CAD build for the part. Positions are in the model's coordinates, mm. A direction names the side the tool comes from. Give positions to 0.01 mm unless a question says otherwise; leave off trailing zeros. Order: outer loops, then holes, each group sorted by start corner. A loop starts at its lowest first (then second) coordinate and runs counter-clockwise, first axis right, second up. Notation, with made-up numbers: M 80,80.5 L 133,80.5 A33 ccw 133,118.5 Z; hole C 31.5,50 d3. An arc over 180 degrees is marked long. Put each result on its own line as item: value. Start each with the question number.
1) Cut at B-B (y = -32). Write the cut outline in (x, z).
2) Cut at C-C (x = 6). Write the cut outline in (y, z), and give its area (3 significant figures).
3) Drill centre lines: line 1 (Y direction, x = 0, z = 1.6); line 2 (Y direction, x = 0, z = 6.45); line 3 (Y direction, x = -38.9, z = 3.6). Where is each one in solid material? Low to high. Write a range as [from, to].
4) Two-plate mould, pull along Z, no slides. Class faces 1 (the face through (-19.43, 0.22, 11.4)), 2 (the face through (-20.6, 0.32, 8.57)), 3 (the face through (0, -34, 2)): released by +Z, released by -Z, zero draft, split by the parting line, or undercut.
5) Cut at A-A (x = 38.9). Write the cut outline in (y, z), and give its area (3 significant figures).
6) Pin check, flat tips, straight feed: pin 1 (1.5 mm diameter, centred on y = -9.5, z = 20, fed in from +X); pin 2 (7.5 mm diameter, centred on x = -1.5, y = 0, fed in from -Z); pin 3 (10.5 mm diameter, centred on x = 0, y = -32, fed in from +Z); pin 4 (9 mm diameter, centred on x = 0.5, y = -30.5, fed in from +Z). Stop position of each tip, or through.
7) Tool access for faces 4 (the face through (0, 25, 15)), 5 (the face through (-10, 0, 22)), 6 (the face through (-1.708, -3.015, 2.465)): list every direction of +Z, -Z, +X, -X, +Y, -Y with a clear straight run to the whole face (end or side of a thin tool).
8) Cut at D-D (x = -24). Write the cut outline in (y, z), and give its area (3 significant figures).
```python
from build123d import *

# Parameters (mm, degrees)
SKETCH1_W           = 93.8
SKETCH1_H           = 80
BOSS_EXTRUDE1_DEPTH = 8
SKETCH2_W           = 40
SKETCH2_H           = 50
BOSS_EXTRUDE2_DEPTH = 15
SKETCH4_R           = 2
CUT_EXTRUDE2_DEPTH  = 66.792172787
CUT_EXTRUDE3_DEPTH  = 5
SKETCH7_R           = 2
CUT_EXTRUDE4_DEPTH  = 20
SKETCH8_R           = 4
CUT_EXTRUDE5_DEPTH  = 3
CUT_EXTRUDE6_DEPTH  = 82.268751682
SKETCH10_W          = 3
SKETCH10_H          = 50
CUT_EXTRUDE7_DEPTH  = 2
FILLET2_R           = 2


with BuildPart() as part:
    # Sketch1 → Boss-Extrude1 (new body)
    with BuildSketch(Plane.XY):
        Rectangle(SKETCH1_W, SKETCH1_H)
    extrude(amount=BOSS_EXTRUDE1_DEPTH)

    # Sketch2 → Boss-Extrude2 (add)
    with BuildSketch(Plane.XY.offset(8)):
        Rectangle(SKETCH2_W, SKETCH2_H)
    extrude(amount=BOSS_EXTRUDE2_DEPTH)

    # Sketch4 → Cut-Extrude2 (cut, through all)
    with BuildSketch(Plane(origin=(0, 0, 0), x_dir=(-1, 0, 0), z_dir=(0, 0, -1))):
        with Locations((0, -32)):
            Circle(SKETCH4_R)
        with Locations((0, 32)):
            Circle(SKETCH4_R)
        with Locations((38.9, 0)):
            Circle(SKETCH4_R)
        with Locations((-38.9, 0)):
            Circle(SKETCH4_R)
    extrude(amount=-CUT_EXTRUDE2_DEPTH, mode=Mode.SUBTRACT)

    # Sketch5 → Cut-Extrude3 (cut)
    with BuildSketch(Plane(origin=(0, 0, 0), x_dir=(-1, 0, 0), z_dir=(0, 0, -1))):
        Polygon((0, 4.001037365), (-3.465, 2.000518683), (-3.465, -2.000518683), (0, -4.001037365), (3.465, -2.000518683), (3.465, 2.000518683), align=None)
    extrude(amount=-CUT_EXTRUDE3_DEPTH, mode=Mode.SUBTRACT)

    # Sketch7 → Cut-Extrude4 (cut)
    with BuildSketch(Plane(origin=(0, 0, 5), x_dir=(-1, 0, 0), z_dir=(0, 0, -1))):
        Circle(SKETCH7_R)
    extrude(amount=-CUT_EXTRUDE4_DEPTH, mode=Mode.SUBTRACT)

    # Sketch8 → Cut-Extrude5 (cut)
    with BuildSketch(Plane.XY.offset(8)):
        with Locations((0, 32)):
            Circle(SKETCH8_R)
        with Locations((38.9, 0)):
            Circle(SKETCH8_R)
        with Locations((0, -32)):
            Circle(SKETCH8_R)
        with Locations((-38.9, 0)):
            Circle(SKETCH8_R)
    extrude(amount=-CUT_EXTRUDE5_DEPTH, mode=Mode.SUBTRACT)

    # Sketch9 → Cut-Extrude6 (cut, through all)
    with BuildSketch(Plane(origin=(20, 0, 0), x_dir=(0, 0, -1), z_dir=(1, 0, 0))):
        with BuildLine():
            Line((-12, 16), (-12, -16))
            ThreePointArc((-12, -16), (-15.5, -19.5), (-19, -16))
            Line((-19, -16), (-19, 16))
            ThreePointArc((-19, 16), (-15.5, 19.5), (-12, 16))
        make_face()
    extrude(amount=-CUT_EXTRUDE6_DEPTH, mode=Mode.SUBTRACT)

    # Sketch10 → Cut-Extrude7 (cut)
    with BuildSketch(Plane.XY.offset(23)):
        with Locations((-11.5, 0)):
            Rectangle(SKETCH10_W, SKETCH10_H)
        with Locations((11.5, 0)):
            Rectangle(SKETCH10_W, SKETCH10_H)
    extrude(amount=-CUT_EXTRUDE7_DEPTH, mode=Mode.SUBTRACT)

    # Fillet2
    fillet2_edges = [part.edges().sort_by_distance(p)[0] for p in [
        (20, 0, 23),
        (20, 0, 8),
        (20, -19.5, 15.5),
        (20, 0, 12),
        (20, 19.5, 15.5),
        (20, 0, 19),
        (0, 25, 8),
        (20, 25, 15.5),
        (16.5, 25, 23),
        (13, 25, 22),
        (11.5, 25, 21),
        (10, 25, 22),
        (0, 25, 23),
        (-10, 25, 22),
        (-11.5, 25, 21),
        (-13, 25, 22),
        (-16.5, 25, 23),
        (-20, 25, 15.5),
        (-20, 0, 23),
        (-20, 0, 8),
        (-20, -19.5, 15.5),
        (-20, 0, 19),
        (-20, 19.5, 15.5),
        (-20, 0, 12),
        (-10, -25, 22),
        (0, -25, 23),
        (10, -25, 22),
        (11.5, -25, 21),
        (13, -25, 22),
        (16.5, -25, 23),
        (20, -25, 15.5),
        (0, -25, 8),
        (-20, -25, 15.5),
        (-16.5, -25, 23),
        (-13, -25, 22),
        (-11.5, -25, 21),
    ]]
    fillet(fillet2_edges, radius=FILLET2_R - 0.0001)  # a hair under: the kernel refuses the full size


solid = part.part
```
Solution:
1. outline: M -46.9,0 L -2,0 L -2,5 L -4,5 L -4,8 L -46.9,8 Z; M 2,0 L 46.9,0 L 46.9,8 L 4,8 L 4,5 L 2,5 Z
2. outline: M -40,0 L 40,0 L 40,8 L 27,8 A2 cw 25,10 L 25,21 A2 ccw 23,23 L -23,23 A2 ccw -25,21 L -25,10 A2 cw -27,8 L -40,8 Z; hole M -16,12 L 16,12 A3.5 ccw 16,19 L -16,19 A3.5 ccw Z
2. area: 1,130 mm²
3. line 1: [-40, -34], [-30, -4], [4, 30], [34, 40]
3. line 2: [-40, -36], [-28, -2], [2, 28], [36, 40]
3. line 3: [-40, -2], [2, 40]
4. face 1: undercut
4. face 2: released by +Z
4. face 3: zero draft
5. outline: M -40,0 L -2,0 L -2,5 L -4,5 L -4,8 L -40,8 Z; M 2,0 L 40,0 L 40,8 L 4,8 L 4,5 L 2,5 Z
5. area: 596 mm²
6. pin 1: x = 19.98
6. pin 2: z = 0
6. pin 3: z = 8.02
6. pin 4: z = 8.27
7. face 4: +Z, +X, -X, +Y
7. face 5: +Z, +Y, -Y
7. face 6: -Z
8. outline: M -40,0 L 40,0 L 40,8 L -40,8 Z
8. area: 640 mm²
